Autodesk Inventor part; units mm, degrees
ref_plane "Work Plane1" through (0, 0, 42.78) normal (0, 0, 1) x (1, 0, 0)
ref_plane "YZ Plane" through (0, 0, 0) normal (1, 0, 0) x (0, 1, 0)
ref_plane "XZ Plane" through (0, 0, 0) normal (0, 1, 0) x (-1, 0, 0)
sketch "Sketch1" plane through (0, 0, 0) normal (0, 0, 1) x (1, 0, 0)
  circle A0 centre (0, 0) radius 5
  dimension "d0" = 10
extrude "Extrusion1" add sketch "Sketch1" along normal blind 12.7
sketch "Sketch2" plane through (0, 0, 12.7) normal (0, 0, 1) x (1, 0, 0)
  point P0 (0, 0)
thread "Thread1"
ref_plane "Work Plane1" through (0, 0, 42.78) normal (0, 0, 1) x (1, 0, 0)
sketch "Sketch3" plane through (0, 0, 42.78) normal (0, 0, 1) x (1, 0, 0)
  circle A0 centre (0, 0) radius 5
extrude "Extrusion2" add sketch "Sketch3" along normal blind 12.7
thread "Thread2"
sketch "Sketch4" plane through (0, 0, 42.78) normal (0, 0, -1) x (-1, 0, 0)
  circle A0 centre (0, 0) radius 5
extrude "Extrusion3" add sketch "Sketch4" along normal blind 30.08
sketch "Sketch5" plane through (0, 0, 55.48) normal (0, 0, 1) x (1, 0, 0)
  line L0 (-0.635, 2.54) -> (0.635, 2.54)
  line L1 (0.635, 2.54) -> (0.635, -2.54)
  line L2 (0.635, -2.54) -> (-0.635, -2.54)
  line L3 (-0.635, -2.54) -> (-0.635, 2.54)
  line L4 (-0.635, 2.54) -> (0.635, -2.54) construction
  line L5 (0.635, 2.54) -> (-0.635, -2.54) construction
  point P0 (0, 0)
  dimension "d15" = 1.27
  dimension "d16" = 5.08
extrude "Extrusion4" cut sketch "Sketch5" against normal through all
properties part number "Pedal Axle"
The model under review builds one solid part; all positions refer to its coordinate system, in mm. A direction names the side the tool comes from. Give positions to 0.01 mm unless a question says otherwise; leave off trailing zeros. Write each loop counter-clockwise with the first axis right and the second up, starting at its lowest first coordinate (ties: lowest second). Pieces come first, ordered by that corner, then holes. Notation, with made-up numbers: (89, -11.5) -> (123, -11.5) arc R24 ccw to (123, -0.5) -> close; hole circle Ø4 at (84, 14.25). An arc over 180 degrees is marked (long way). Put each result on its own line as item: value.
(1) For pin 1 Ø1.5 at (x, z) = (-3, 19) entering from -Y, flat-tipped, find the tip position at first contact; note if it passes through.
Results are:
pin 1: y = -4.47
(2) The part is to be moulded in two halves that separate along Y. For faces 3 (the flat face through (-0.635, 0, 28)), 4 (the flat face through (1, 0, 0)), 5 (the flat face through (0.635, 0, 28)), say which applies: pulls with the +Y half, pulls with the -Y half, needs draft (parallel to the pull), parting line crosses it, or undercut.
Results are:
face 3: undercut
face 4: needs draft
face 5: undercut
(3) We need section D-D, the plane y = 4. Give the boundary of the cut face in (x, z), and give its area (3 significant figures).
Results are:
outline: (-3, 0) -> (3, 0) -> (3, 55.48) -> (-3, 55.48) -> close
area: 333 mm²
(4) Tool access review of faces 1 (the flat face through (0, 2.54, 28)), 2 (the flat face through (1, 0, 55.48)): name each direction out of +Z, -Z, +X, -X, +Y, -Y from which nothing blocks a thin tool from reaching the whole face with its end or side.
Results are:
face 1: +Z, -Z
face 2: +Z, +X, -X, +Y, -Y
(5) We need section C-C, the plane z = 15.5. Give the boundary of the cut face in (x, y) (3 decimals), and give its area (3 significant figures).
Results are:
outline: circle Ø10 at (0, 0); hole (-0.635, -2.54) -> (0.635, -2.54) -> (0.635, 2.54) -> (-0.635, 2.54) -> close
area: 72.1 mm²
(6) We need section B-B, the plane y = 0. Give the boundary of the cut face in (x, z) (3 decimals), and give its area (3 significant figures).
Results are:
outline: (-5, 0) -> (-0.635, 0) -> (-0.635, 55.48) -> (-5, 55.48) -> close; (0.635, 0) -> (5, 0) -> (5, 55.48) -> (0.635, 55.48) -> close
area: 484 mm²
(7) To check wall thickness, follow probe 1 along Y at (x, z) = (0, 27); probe 2 along X at (y, z) = (-0.25, 15) (3 decimals); probe 3 along X at (y, z) = (1.25, 27.5) (3 decimals). State the ranges of each line that lie inside material, in increasing order. Write a range as from..to.
Results are:
probe 1: -5..-2.54, 2.54..5
probe 2: -4.994..-0.635, 0.635..4.994
probe 3: -4.841..-0.635, 0.635..4.841
(8) We need section A-A, the plane x = 0. Give the boundary of the cut face in (y, z).
Results are:
outline: (-5, 0) -> (-2.54, 0) -> (-2.54, 55.48) -> (-5, 55.48) -> close; (2.54, 0) -> (5, 0) -> (5, 55.48) -> (2.54, 55.48) -> close
